```python
from build123d import *

# Parameters (mm, degrees)
SKETCH_R        = 25
PAD_DEPTH       = 35
SKETCH001_W     = 50
SKETCH001_H     = 40
PAD001_DEPTH    = 31
SKETCH002_W     = 34
SKETCH002_H     = 67.560009
POCKET_DEPTH    = 50.001
SKETCH003_R     = 16
POCKET001_DEPTH = 70.001
SKETCH004_W     = 40
SKETCH004_H     = 50
PAD002_DEPTH    = 70
SKETCH005_R     = 25
PAD003_DEPTH    = 23
SKETCH007_W     = 30
SKETCH007_H     = 36
PAD005_DEPTH    = 21
SKETCH006_R     = 18
PAD004_DEPTH    = 24
SKETCH008_W     = 18
SKETCH008_H     = 51.791633
POCKET002_DEPTH = 36.001
SKETCH009_R     = 7.5
POCKET003_DEPTH = 36.001
SKETCH010_W     = 57
SKETCH010_H     = 36
PAD006_DEPTH    = 9
SKETCH011_R     = 12.5
POCKET004_DEPTH = 58.001
SKETCH012_R     = 7.5
POCKET005_DEPTH = 59.001


with BuildPart() as pad:
    # Sketch → Pad (new body, symmetric)
    with BuildSketch(Plane.YZ):
        Circle(SKETCH_R)
    extrude(amount=PAD_DEPTH, both=True)


with BuildPart() as pad002:
    # Sketch001 → Pad001 (new body, symmetric)
    with BuildSketch(Plane.YZ):
        with Locations((0, 20)):
            Rectangle(SKETCH001_W, SKETCH001_H)
    extrude(amount=PAD001_DEPTH, both=True)

    # Fusion: union Pad
    add(pad.part)

    # Sketch002 → Pocket (cut, through all)
    with BuildSketch(Plane.XZ.offset(25)):
        with Locations((1.376189, -5.780005)):
            Rectangle(SKETCH002_W, SKETCH002_H)
    extrude(amount=-POCKET_DEPTH, mode=Mode.SUBTRACT)

    # Sketch003 → Pocket001 (cut, through all)
    with BuildSketch(Plane.YZ.offset(35)):
        Circle(SKETCH003_R)
    extrude(amount=-POCKET001_DEPTH, mode=Mode.SUBTRACT)

    # Sketch004 → Pad002 (new body)
    with BuildSketch(Plane.XY.offset(40)):
        Rectangle(SKETCH004_W, SKETCH004_H)
    extrude(amount=PAD002_DEPTH)


with BuildPart() as fusion003:
    # Sketch005 → Pad003 (new body, symmetric)
    with BuildSketch(Plane.YZ):
        with Locations((0, 110)):
            Circle(SKETCH005_R)
    extrude(amount=PAD003_DEPTH, both=True)

    # Fusion003: union Pad002
    add(pad002.part)


with BuildPart() as pad005:
    # Sketch007 → Pad005 (new body, symmetric)
    with BuildSketch(Plane.YZ):
        with Locations((-70, 115)):
            Rectangle(SKETCH007_W, SKETCH007_H)
    extrude(amount=PAD005_DEPTH, both=True)


with BuildPart() as pocket003:
    # Sketch006 → Pad004 (new body, symmetric)
    with BuildSketch(Plane.YZ):
        with Locations((-85, 115)):
            Circle(SKETCH006_R)
    extrude(amount=PAD004_DEPTH, both=True)

    # Fusion001: union Pad005
    add(pad005.part)

    # Sketch008 → Pocket002 (cut, through all)
    with BuildSketch(Plane.XY.offset(133)):
        with Locations((0, -92.895816)):
            Rectangle(SKETCH008_W, SKETCH008_H)
    extrude(amount=-POCKET002_DEPTH, mode=Mode.SUBTRACT)

    # Sketch009 → Pocket003 (cut, through all)
    with BuildSketch(Plane.XY.offset(133)):
        with Locations((-85, 110)):
            Circle(SKETCH009_R)
    extrude(amount=-POCKET003_DEPTH, mode=Mode.SUBTRACT)


with BuildPart() as pocket005:
    # Sketch010 → Pad006 (new body, symmetric)
    with BuildSketch(Plane.YZ):
        with Locations((-28.5, 115)):
            Rectangle(SKETCH010_W, SKETCH010_H)
    extrude(amount=PAD006_DEPTH, both=True)

    # Fusion002: union Pocket003
    add(pocket003.part)

    # Fusion004: union Fusion003
    add(fusion003.part)

    # Sketch011 → Pocket004 (cut, through all)
    with BuildSketch(Plane.YZ.offset(23)):
        with Locations((0, 110)):
            Circle(SKETCH011_R)
    extrude(amount=-POCKET004_DEPTH, mode=Mode.SUBTRACT)

    # Sketch012 → Pocket005 (cut, through all)
    with BuildSketch(Plane.YZ.offset(24)):
        with Locations((-85, 115)):
            Circle(SKETCH012_R)
    extrude(amount=-POCKET005_DEPTH, mode=Mode.SUBTRACT)


solid = pocket005.part
```
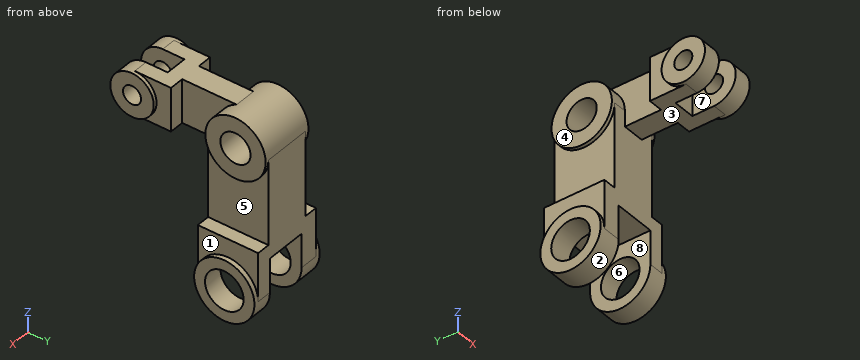
Design review of the part built by this model. Coordinates are the model's own, in mm. Face numbers are marked on the shaded views. A direction names the side the tool comes from. Round coordinates to 2 decimals unless told otherwise and drop trailing zeros. Write each loop counter-clockwise with the first axis right and the second up, starting at its lowest first coordinate (ties: lowest second). Pieces come first, ordered by that corner, then holes. Notation, with made-up numbers: (64, -31.75) -> (80, -31.75) arc R24 cw to (80, -3.75) -> close; hole circle Ø1 at (11, 71.5). An arc over 180 degrees is marked (long way). Answer in a Markdown table with one row per item.
Q1. Take a section at D-D, the plane z = 75.5. State the section outline as (x, y) points, then the cut area to 3 significant figures.
The answers:
| item | result |
|---|---|
| outline | (-20, -25) -> (20, -25) -> (20, 25) -> (-20, 25) -> close |
| area | 2,000 mm² |
Q2. For the marked faces 1, 2, 3 and 4, list the 3-axis set-ups (+Z, -Z, +X, -X, +Y, -Y) from which the entire face can be reached by the end or side of a thin tool; tool diameter is ignored.
The answers:
| item | result |
|---|---|
| face 1 | +Z, +X |
| face 2 | -X |
| face 3 | -Z, +X, -X, -Y |
| face 4 | +Z, -X, +Y |
Q3. Take a section at C-C, the plane y = -94.5. State the section outline as (x, z) points, then the cut area to 3 significant figures.
The answers:
| item | result |
|---|---|
| outline | (-24, 99.71) -> (-9, 99.71) -> (-9, 130.29) -> (-24, 130.29) -> close; (9, 99.71) -> (24, 99.71) -> (24, 130.29) -> (9, 130.29) -> close |
| area | 917 mm² |
Q4. Clearance check with flat-ended pins moving along their axes: pin 1 Ø15 at (y, z) = (-12, 58) entering from -X; pin 2 Ø2 at (x, y) = (17, -67) entering from +Z; pin 3 Ø21 at (x, y) = (1, -42.5) entering from -Z; pin 4 Ø20 at (y, z) = (9, 10.5) entering from -X. State where each tip first meets the part, or that it passes through.
The answers:
| item | result |
|---|---|
| pin 1 | x = -20 |
| pin 2 | z = 133 |
| pin 3 | z = 97 |
| pin 4 | x = -35 |
Q5. Take a section at A-A, the plane y = 0. Count the separate pieces of the cut face and the enclosed holes in it, then the cut area to 3 significant figures.
The answers:
| item | result |
|---|---|
| separate pieces | 4 |
| enclosed holes | 0 |
| area | 4,430 mm² |
Q6. To check wall thickness, follow L1, parallel to Z at x = -1, y = 0; L2, parallel to X at y = -76.5, z = 112; L3, parallel to Z at x = 19, y = -85. State the ranges of each line that lie inside material, in increasing order. Write a range as [from, to].
The answers:
| item | result |
|---|---|
| L1 | [28, 97.5], [122.5, 135] |
| L2 | [-24, -9], [9, 24] |
| L3 | [97, 107.5], [122.5, 133] |
Q7. Draft analysis for pull direction X (two halves, no side actions). For the marked faces 5, 6, 7 and 8, state which applies: +X half, -X half, draft (parallel to the pull), parting line (faces both ways), or undercut.
The answers:
| item | result |
|---|---|
| face 5 | +X half |
| face 6 | draft |
| face 7 | undercut |
| face 8 | undercut |
